The model under review builds one solid part; all positions refer to its coordinate system, in mm. Face numbers are marked on the shaded views. Round coordinates to 2 decimals unless told otherwise and drop trailing zeros. Write each loop counter-clockwise with the first axis right and the second up, starting at its lowest first coordinate (ties: lowest second). Pieces come first, ordered by that corner, then holes.
Item 1: To check wall thickness, follow L1, parallel to Y at x = 0, z = -17; L2, parallel to Y at x = 1.75, z = 12; L3, parallel to X at y = -0.5, z = -21.5. State the ranges of each line that lie inside material, in increasing order.
Item 2: Add section A-A (z = -14). Give the boundary of the cut face in (x, y).
Item 3: Add section B-B (x = 0). Give the boundary of the cut face in (y, z) (3 decimals), plus the area to 3 significant figures.
Item 4: Draft analysis for pull direction Z (two halves, no side actions). For the marked faces 1, 2 and 3, state which applies: +Z half, -Z half, draft (parallel to the pull), parting line (faces both ways), or undercut.
Item 5: Add section C-C (y = 0). Give the boundary of the cut face in (x, z) (3 decimals).
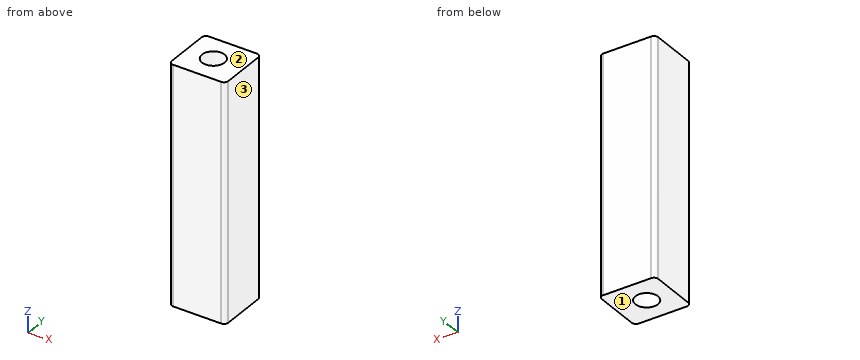
```python
from build123d import *

# Parameters (mm, degrees)
SKETCH1_W           = 12.7
SKETCH1_H           = 12.7
SKETCH1_R           = 2.7
BOSS_EXTRUDE1_DEPTH = 28.275
SKETCH4_W           = 56.55
SKETCH4_H           = 12.7
BOSS_EXTRUDE3_DEPTH = 0.79375
FILLET2_R           = 1


with BuildPart() as part:
    # Sketch1 → Boss-Extrude1 (new, symmetric)
    with BuildSketch(Plane.XY):
        Rectangle(SKETCH1_W, SKETCH1_H)
        Circle(SKETCH1_R, mode=Mode.SUBTRACT)
    extrude(amount=BOSS_EXTRUDE1_DEPTH, both=True)

    # Sketch4 → Boss-Extrude3 (add)
    with BuildSketch(Plane(origin=(6.35, 0, 0), x_dir=(0, 0, -1), z_dir=(1, 0, 0))):
        Rectangle(SKETCH4_W, SKETCH4_H)
    extrude(amount=BOSS_EXTRUDE3_DEPTH)

    # Fillet2
    fillet2_edges = [part.edges().sort_by_distance(p)[0] for p in [
        (7.14375, -6.35, 0),
        (7.14375, 6.35, 0),
        (-6.35, -6.35, 0),
        (-6.35, 6.35, 0),
    ]]
    fillet(fillet2_edges, radius=FILLET2_R)


solid = part.part
```
Numbers:
1. L1: y = -6.35 to -2.7, 2.7 to 6.35
1. L2: y = -6.35 to -2.06, 2.06 to 6.35
1. L3: x = -6.35 to -2.65, 2.65 to 7.14
2. outline: (-6.35, -5.35) arc R1 ccw to (-5.35, -6.35) - (6.14, -6.35) arc R1 ccw to (7.14, -5.35) - (7.14, 5.35) arc R1 ccw to (6.14, 6.35) - (-5.35, 6.35) arc R1 ccw to (-6.35, 5.35) - close; hole circle Ø5.4 at (0, 0)
3. outline: (-6.35, -28.275) - (-2.7, -28.275) - (-2.7, 28.275) - (-6.35, 28.275) - close; (2.7, -28.275) - (6.35, -28.275) - (6.35, 28.275) - (2.7, 28.275) - close
3. area: 413 mm2
4. face 1: -Z half
4. face 2: +Z half
4. face 3: draft
5. outline: (-6.35, -28.275) - (-2.7, -28.275) - (-2.7, 28.275) - (-6.35, 28.275) - close; (2.7, -28.275) - (7.144, -28.275) - (7.144, 28.275) - (2.7, 28.275) - close
